Work out the finished part from the listing and answer in its coordinate system (mm). A direction names the side the tool comes from. Round coordinates to 2 decimals unless told otherwise and drop trailing zeros. Write each loop counter-clockwise with the first axis right and the second up, starting at its lowest first coordinate (ties: lowest second). Pieces come first, ordered by that corner, then holes. Notation, with made-up numbers: M 88.25,-3.5 L 107.25,-3.5 A9 ccw 107.25,4.5 Z; hole C -35,26 d8. An arc over 180 degrees is marked long. Answer in a Markdown table with one row per item.
```python
from build123d import *

# Parameters (mm, degrees)
DRAFT1_ANGLE = 0.5
FILLET2_R    = 1


with BuildPart() as part:
    # Sketch1 → Revolve1 (revolve)
    with BuildSketch(Plane.XY, mode=Mode.PRIVATE) as revolve1_sk:
        Polygon((0, 0), (5, 0), (5, 4), (20, 4), (20, 7), (0, 7), align=None)
    revolve(revolve1_sk.sketch.rotate(Axis((-15.220779221, -4, 0), (1, 0, 0)), 90), axis=Axis((-15.220779221, -4, 0), (1, 0, 0)))

    # Draft1
    draft1_faces = [part.faces().sort_by_distance(p)[0] for p in [
        (12.5, -4, -8),
    ]]
    draft(draft1_faces, Plane(origin=(5, 0, 0), x_dir=(0, 0, 1), z_dir=(1, 0, 0)), DRAFT1_ANGLE)

    # Fillet2
    fillet2_edges = [part.edges().sort_by_distance(p)[0] for p in [
        (20, -4, -8.130903017),
    ]]
    fillet(fillet2_edges, radius=FILLET2_R)


solid = part.part
```
1. Given pin 1 (8 mm diameter, centred on y = -2, z = -1.5, fed in from +X); pin 2 (3 mm diameter, centred on x = 17, y = -8, fed in from -Z); pin 3 (8 mm diameter, centred on x = 14.5, z = 7.5, fed in from -Y); pin 4 (10 mm diameter, centred on y = -8.5, z = -3, fed in from -X), each flat-ended and moving along its own axis, determine where each tip first touches the part or whether it passes through.
Calculated:
| item | result |
|---|---|
| pin 1 | stops at x = 5 |
| pin 2 | stops at z = -10.71 |
| pin 3 | stops at y = -14.43 |
| pin 4 | stops at x = 0 |
2. Determine the mould class of faces 3 (the cylindrical face through (9.86, 6.74, -2.38)), 4 (the cylindrical face through (2.535, -0.095, -0.867)), 5 (the flat face through (0, 1, 0)) for opening direction Y: released by +Y, released by -Y, zero draft, split by the parting line, or undercut.
Calculated:
| item | result |
|---|---|
| face 3 | split by the parting line |
| face 4 | undercut |
| face 5 | zero draft |
3. Consider line 1 along Y through (x, z) = (2.6, 0); line 2 along Z through (x, y) = (7.25, -2.25); line 3 along Y through (x, z) = (3.75, 0.75). Determine where each line is inside the solid, lowest interval first. Write a range as from..to.
Calculated:
| item | result |
|---|---|
| line 1 | y = -15..-8, 0..7 |
| line 2 | z = -10.86..-7.83, 7.83..10.86 |
| line 3 | y = -14.97..-7.93, -0.07..6.97 |
4. A tool of negligible diameter and unlimited length cuts with its end or side. For faces 1 (the flat face through (5, -8, -2)), 2 (the flat face through (20, -11, 7)), from which of +Z, -Z, +X, -X, +Y, -Y can it reach the whole face along a straight path? Write none if from no direction.
Calculated:
| item | result |
|---|---|
| face 1 | +X |
| face 2 | +Z, -Z, +X, +Y, -Y |
5. The part is cut by section A-A (x = 2). Determine the outline of the cut face in (y, z), plus the area to 3 significant figures.
Calculated:
| item | result |
|---|---|
| outline | C -4,0 d22; hole C -4,0 d8 |
| area | 330 mm² |
